The figure shows three views and two pictorial views of one solid part (mm, origin at its lowest corner). Answer the questions. Coordinates: 2 decimals unless noted, no trailing zeros. Write each loop counter-clockwise with the first axis right and the second up, starting at its lowest first coordinate (ties: lowest second). Pieces come first, ordered by that corner, then holes. Notation, with made-up numbers: M 32,-12 L 49,-12 A11 cw 49,-1 Z; hole C -8,0 d9. An arc over 180 degrees is marked long. Use CSV: the item, a comma, the result in double quotes.
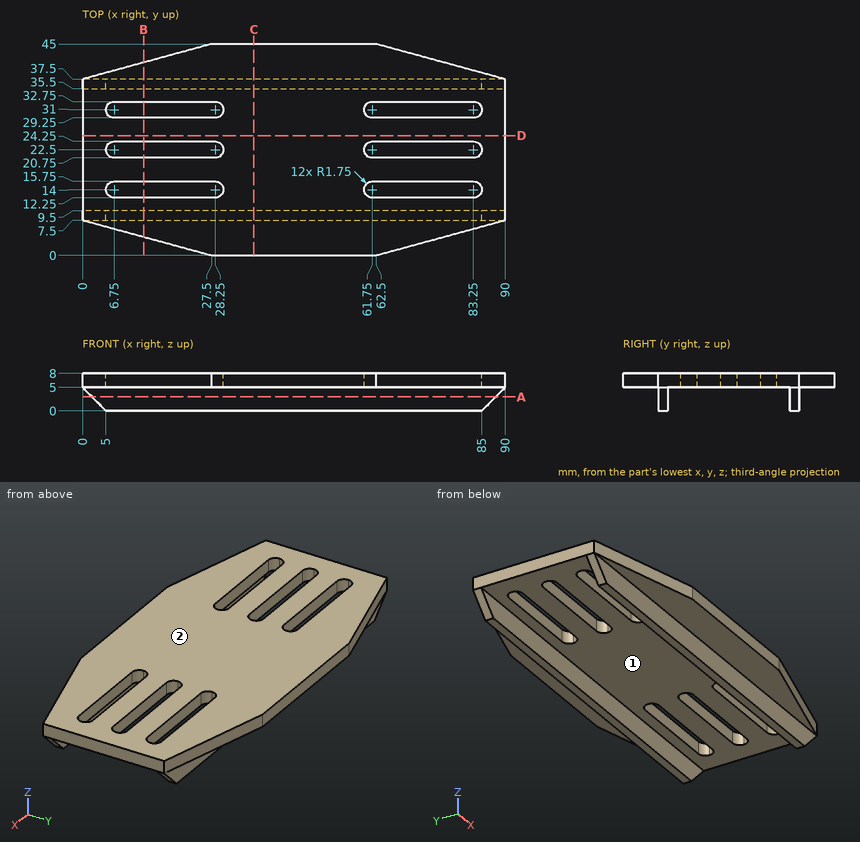
Item 1: The part is cut by section C-C (x = 36.5). Write down the section's boundary in (y, z).
Answer:
outline,"M 0,5 L 7.5,5 L 7.5,0 L 9.5,0 L 9.5,5 L 35.5,5 L 35.5,0 L 37.5,0 L 37.5,5 L 45,5 L 45,8 L 0,8 Z"
Item 2: The part is cut by section A-A (z = 3). Write down the section's boundary in (x, y), then the cut area to 3 significant figures.
Answer:
outline,"M 2,7.5 L 88,7.5 L 88,9.5 L 2,9.5 Z; M 2,35.5 L 88,35.5 L 88,37.5 L 2,37.5 Z"
area,"344 mm2"
Item 3: The part is cut by section B-B (x = 13). Write down the section's boundary in (y, z), then the cut area to 3 significant figures.
Answer:
outline,"M 3.95,5 L 7.5,5 L 7.5,0 L 9.5,0 L 9.5,5 L 12.25,5 L 12.25,8 L 3.95,8 Z; M 15.75,5 L 20.75,5 L 20.75,8 L 15.75,8 Z; M 24.25,5 L 29.25,5 L 29.25,8 L 24.25,8 Z; M 32.75,5 L 35.5,5 L 35.5,0 L 37.5,0 L 37.5,5 L 41.05,5 L 41.05,8 L 32.75,8 Z"
area,"99.8 mm2"
Item 4: Given pin 1 (0.9 mm diameter, centred on x = 71.5, z = 7, fed in from +Y); pin 2 (1.5 mm diameter, centred on x = 17, z = 7, fed in from -Y); pin 3 (1.5 mm diameter, centred on x = 22.5, z = 7, fed in from +Y); pin 4 (8 mm diameter, centred on x = 45, y = 34, fed in from -Z), each flat-ended and moving along its own axis, determine where each tip first touches the part or whether it passes through.
Answer:
pin 1,"stops at y = 42.67"
pin 2,"stops at y = 2.66"
pin 3,"stops at y = 43.84"
pin 4,"stops at z = 0"
Item 5: The part is cut by section D-D (y = 25.5). Write down the section's boundary in (x, z), then the cut area to 3 significant figures.
Answer:
outline,"M 0,5 L 90,5 L 90,8 L 0,8 Z"
area,"270 mm2"
Item 6: Consider probe 1 along Y at (x, z) = (35, 1.25); probe 2 along Z at (x, y) = (22.5, 7); probe 3 along X at (y, z) = (23, 6). Determine where each line is inside the solid, lowest interval first.
Answer:
probe 1,"y = 7.5 to 9.5, 35.5 to 37.5"
probe 2,"z = 5 to 8"
probe 3,"x = 0 to 5.07, 29.93 to 60.07, 84.93 to 90"
Item 7: For a pull along Y with two mould halves and no side action, classify the marked faces 1 and 2 as released by +Y, released by -Y, zero draft, split by the parting line, or undercut.
Answer:
face 1,"undercut"
face 2,"zero draft"
